from build123d import *

# Parameters (mm, degrees)
SKETCH1_R           = 38.1
BOSS_EXTRUDE1_DEPTH = 6.35
SKETCH4_R           = 3.175
CUT_EXTRUDE2_DEPTH  = 55.254423783
SKETCH2_R           = 2.38125
CUT_EXTRUDE3_DEPTH  = 55.254423783


with BuildPart() as part:
    # Sketch1 → Boss-Extrude1 (new body)
    with BuildSketch(Plane.XY):
        Circle(SKETCH1_R)
    extrude(amount=BOSS_EXTRUDE1_DEPTH)

    # Sketch4 → Cut-Extrude2 (cut, through all)
    with BuildSketch(Plane(origin=(0, 0, 0), x_dir=(-1, 0, 0), z_dir=(0, 0, -1))):
        with Locations((-25.4, 0)):
            Circle(SKETCH4_R)
        with Locations((-12.7, 21.997045256)):
            Circle(SKETCH4_R)
        with Locations((12.7, 21.997045256)):
            Circle(SKETCH4_R)
        with Locations((25.4, 0)):
            Circle(SKETCH4_R)
        with Locations((12.7, -21.997045256)):
            Circle(SKETCH4_R)
        with Locations((-12.7, -21.997045256)):
            Circle(SKETCH4_R)
    extrude(amount=-CUT_EXTRUDE2_DEPTH, mode=Mode.SUBTRACT)

    # Sketch2 → Cut-Extrude3 (cut, through all)
    with BuildSketch(Plane.XY.offset(6.35)):
        Circle(SKETCH2_R)
    extrude(amount=-CUT_EXTRUDE3_DEPTH, mode=Mode.SUBTRACT)


solid = part.part
Geometry: final body of the model. Coordinates: model frame, mm. Give positions to 0.01 mm unless a question says otherwise; leave off trailing zeros. Write each loop counter-clockwise with the first axis right and the second up, starting at its lowest first coordinate (ties: lowest second). Pieces come first, ordered by that corner, then holes. Notation, with made-up numbers: (43.5, 21) - (62.5, 21) arc R11 ccw to (62.5, 34) - close; hole circle Ø4 at (62, 40.25). An arc over 180 degrees is marked (long way). Return JSON: item names as keys, results as strings. Group by question number.
1) Section A-A on y = 0. Return the cut outline in (x, z) (3 decimals), plus the area to 3 significant figures.
2) Section D-D on z = 1.5. State how many separate pieces and enclosed holes the cut face has, plus the area to 3 significant figures.
3) Line query: line 1 (Y direction, x = 12.7, z = 4.5); line 2 (X direction, y = 21.5, z = 2.25); line 3 (Y direction, x = 25.4, z = 3.5) (3 decimals). Output: solid intervals per line, ascending.
4) Section B-B on x = -1.5. Return the cut outline in (y, z), plus the area to 3 significant figures.
5) Section C-C on x = 12.7. Return the cut outline in (y, z).
6) Mould query, pull axis X, two halves, no side actions, for faces 1 (the cylindrical face through (-30.235, -23.183, 3.131)), 2 (the flat face through (8, 1, 6.35)), 3 (the cylindrical face through (22.37, 0.95, 3.13)). Classes: released by +X, released by -X, zero draft, split by the parting line, or undercut.
7) First-contact query: P1, Ø5.5, axis at x = -12.7, y = -22, coming from the +Z side; P2, Ø3, axis at y = 11, z = 5, coming from the +X side; P3, Ø2, axis at x = 24, z = 2, coming from the +Y side; P4, Ø3, axis at x = 2, z = 3, coming from the -Y side. Flat tips, straight axial feed; report the tip coordinate or a pass-through.
Filled in:
{
 "1": {"outline": "(-38.1, 0) - (-28.575, 0) - (-28.575, 6.35) - (-38.1, 6.35) - close; (-22.225, 0) - (-2.381, 0) - (-2.381, 6.35) - (-22.225, 6.35) - close; (2.381, 0) - (22.225, 0) - (22.225, 6.35) - (2.381, 6.35) - close; (28.575, 0) - (38.1, 0) - (38.1, 6.35) - (28.575, 6.35) - close", "area": "373 mm^2"},
 "2": {"separate pieces": "1", "enclosed holes": "7", "area": "4,350 mm^2"},
 "3": {"line 1": "y = -35.92 to -25.17, -18.82 to 18.82, 25.17 to 35.92", "line 2": "x = -31.45 to -15.84, -9.56 to 9.56, 15.84 to 31.45", "line 3": "y = -28.398 to -3.175, 3.175 to 28.398"},
 "4": {"outline": "(-38.07, 0) - (-1.85, 0) - (-1.85, 6.35) - (-38.07, 6.35) - close; (1.85, 0) - (38.07, 0) - (38.07, 6.35) - (1.85, 6.35) - close", "area": "460 mm^2"},
 "5": {"outline": "(-35.92, 0) - (-25.17, 0) - (-25.17, 6.35) - (-35.92, 6.35) - close; (-18.82, 0) - (18.82, 0) - (18.82, 6.35) - (-18.82, 6.35) - close; (25.17, 0) - (35.92, 0) - (35.92, 6.35) - (25.17, 6.35) - close"},
 "6": {"face 1": "split by the parting line", "face 2": "zero draft", "face 3": "undercut"},
 "7": {"P1": "passes through", "P2": "stops at x = 36.9", "P3": "stops at y = 30.37", "P4": "stops at y = -38.1"}
}
